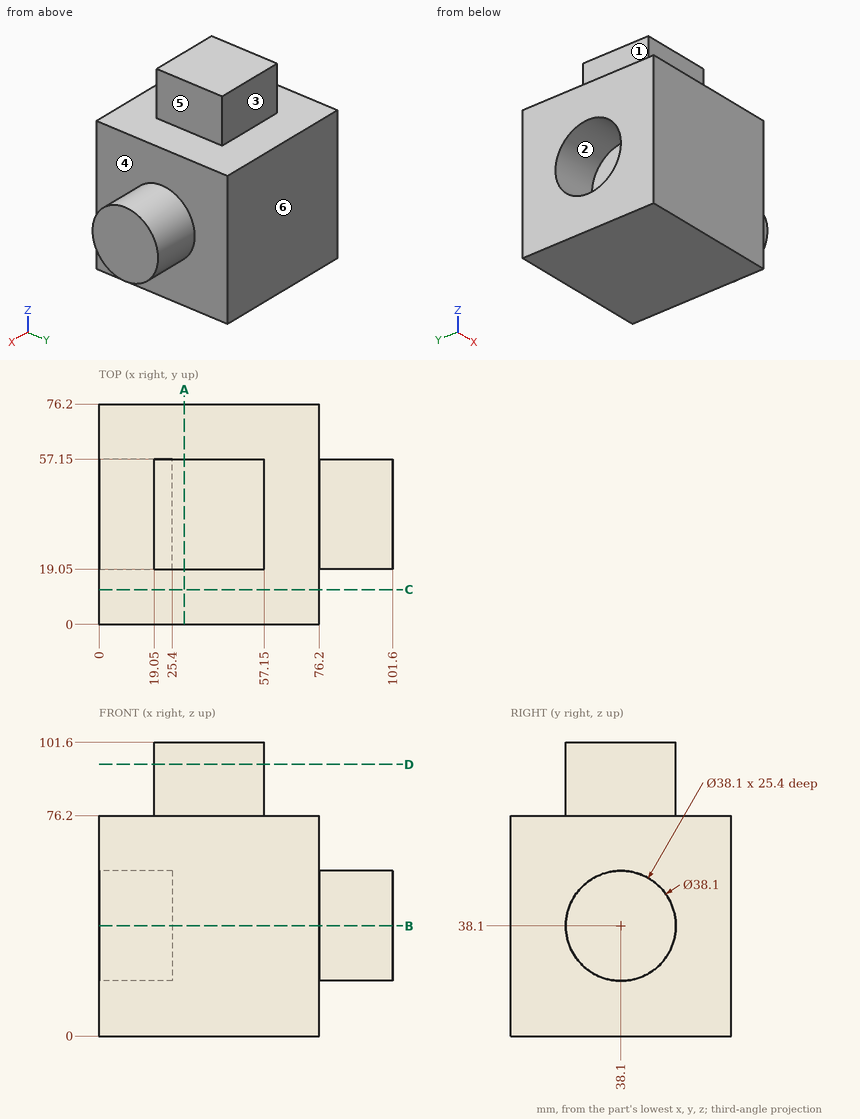
Design review of the part shown in the three views and the two pictorial views. Dimensions are in mm from the part's minimum x, y and z. A direction names the side the tool comes from. Round coordinates to 2 decimals unless told otherwise and drop trailing zeros. Write each loop counter-clockwise with the first axis right and the second up, starting at its lowest first coordinate (ties: lowest second). Pieces come first, ordered by that corner, then holes. Notation, with made-up numbers: (36, 11) - (73, 11) arc R17 ccw to (73, 32) - close; hole circle Ø1 at (20, -28.75). An arc over 180 degrees is marked (long way). Return JSON: item names as keys, results as strings. Group by question number.
Item 1: We need section D-D on z = 94. Write out the cut boundary in (x, y), and give its area (3 significant figures).
Item 2: Insertion check: P1, Ø1.5, axis at y = 57.5, z = 70, coming from the +X side; P2, Ø11.5, axis at y = 34.5, z = 43, coming from the -X side; P3, Ø6, axis at x = 37, z = 86.5, coming from the +Y side. Each pin has a flat end and moves straight along its axis. Give the tip position at first contact, or say it passes through.
Item 3: Machinability: for the marked faces 4, 5 and 6, which of the approach directions +Z, -Z, +X, -X, +Y, -Y give a long, thin tool a straight path to every point of the face, cutting with its end or side? Answer none if there is none.
Item 4: We need section A-A on x = 29.5. Write out the cut boundary in (y, z).
Item 5: We need section C-C on y = 12. Write out the cut boundary in (x, z).
Item 6: For probe 1 along Z at (x, y) = (6.5, 38.1); probe 2 along Z at (x, y) = (50.5, 13.5), list the stretches that pass through material, from the lowest coordinate up. Write a range as [from, to].
Item 7: We need section B-B on z = 38.1. Write out the cut boundary in (x, y).
Item 8: The part is to be moulded in two halves that separate along Y. For the marked faces 1, 2 and 3, say which applies: pulls with the +Y half, pulls with the -Y half, needs draft (parallel to the pull), parting line crosses it, or undercut.
Model answer:
{
 "1": {"outline": "(19.05, 19.05) - (57.15, 19.05) - (57.15, 57.15) - (19.05, 57.15) - close", "area": "1,450 mm²"},
 "2": {"P1": "stops at x = 76.2", "P2": "stops at x = 25.4", "P3": "stops at y = 57.15"},
 "3": {"face 4": "+X", "face 5": "+Z, +X, +Y, -Y", "face 6": "+Z, -Z, +X, -X, +Y"},
 "4": {"outline": "(0, 0) - (76.2, 0) - (76.2, 76.2) - (57.15, 76.2) - (57.15, 101.6) - (19.05, 101.6) - (19.05, 76.2) - (0, 76.2) - close"},
 "5": {"outline": "(0, 0) - (76.2, 0) - (76.2, 76.2) - (0, 76.2) - close"},
 "6": {"probe 1": "z = [0, 19.05], [57.15, 76.2]", "probe 2": "z = [0, 76.2]"},
 "7": {"outline": "(0, 0) - (76.2, 0) - (76.2, 19.05) - (101.6, 19.05) - (101.6, 57.15) - (76.2, 57.15) - (76.2, 76.2) - (0, 76.2) - (0, 57.15) - (25.4, 57.15) - (25.4, 19.05) - (0, 19.05) - close"},
 "8": {"face 1": "needs draft", "face 2": "undercut", "face 3": "pulls with the +Y half"}
}
